from build123d import *

# Parameters (mm, degrees)
BOSS_EXTRUDE1_DEPTH = 15
BOSS_EXTRUDE2_START = 15
BOSS_EXTRUDE2_DEPTH = 3.048
BOSS_EXTRUDE3_START = -15
BOSS_EXTRUDE3_DEPTH = 3.048
SKETCH2_R           = 1.905
CUT_EXTRUDE1_DEPTH  = 46
SKETCH3_R           = 3.5
CUT_EXTRUDE2_DEPTH  = 46


with BuildPart() as part:
    # Sketch1 → Boss-Extrude1 (new, symmetric)
    with BuildSketch(Plane.XY):
        Polygon((-3.048, -30), (0, -30), (0, 0), (-30, 0), (-30, -3.048), (-3.048, -3.048), align=None)
    extrude(amount=BOSS_EXTRUDE1_DEPTH, both=True)

    # Sketch1<3> → Boss-Extrude2 (add)
    with BuildSketch(Plane.XY.offset(BOSS_EXTRUDE2_START)):
        Polygon((-3.048, -30), (-30, -3.048), (-3.048, -3.048), align=None)
    extrude(amount=-BOSS_EXTRUDE2_DEPTH)

    # Sketch1<4> → Boss-Extrude3 (add)
    with BuildSketch(Plane.XY.offset(BOSS_EXTRUDE3_START)):
        Polygon((-3.048, -30), (-30, -3.048), (-3.048, -3.048), align=None)
    extrude(amount=BOSS_EXTRUDE3_DEPTH)

    # Sketch2 → Cut-Extrude1 (cut, through all)
    with BuildSketch(Plane(origin=(0, 0, 0), x_dir=(1, 0, 0), z_dir=(0, 1, 0))):
        with Locations(Location((-15, 0, 0), (0, 0, 270))):
            Circle(SKETCH2_R)
    extrude(amount=-CUT_EXTRUDE1_DEPTH, mode=Mode.SUBTRACT)

    # Sketch3 → Cut-Extrude2 (cut, through all)
    with BuildSketch(Plane(origin=(0, 0, 0), x_dir=(0, 0, -1), z_dir=(1, 0, 0))):
        with Locations((0, -15)):
            Circle(SKETCH3_R)
    extrude(amount=-CUT_EXTRUDE2_DEPTH, mode=Mode.SUBTRACT)


solid = part.part
For this review, take the finished solid that the model builds, in its own axes (mm). A direction names the side the tool comes from. Give positions to 0.01 mm unless a question says otherwise; leave off trailing zeros. Loops run counter-clockwise (first coordinate to the right, second up) from the corner with the lowest first, then second, coordinate; pieces in that order, holes last. Notation, with made-up numbers: (-4.75, -15) -> (11.25, -15) arc R23 cw to (11.25, 19) -> close; hole circle Ø4 at (-21, 64.5). An arc over 180 degrees is marked (long way). One line per question, with ' | ' between items.
1) We need section B-B (y = -12.25). Write out the cut boundary in (x, z), plus the area to 3 significant figures.
Resolved:
outline: (-20.8, -15) -> (0, -15) -> (0, -2.17) -> (-3.05, -2.17) -> (-3.05, -11.95) -> (-20.8, -11.95) -> close; (-20.8, 11.95) -> (-3.05, 11.95) -> (-3.05, 2.17) -> (0, 2.17) -> (0, 15) -> (-20.8, 15) -> close | area: 186 mm2
2) Insertion check: pin 1 Ø12 at (y, z) = (-10.5, -3) entering from -X; pin 2 Ø1 at (x, z) = (-4.5, -4.5) entering from -Y. Each pin has a flat end and moves straight along its axis. Give the tip position at first contact, or say it passes through.
Resolved:
pin 1: stops at x = -3.05 | pin 2: stops at y = -3.05
3) For faces 1 (the flat face through (-16.34, -16.71, 13.5)), 2 (the flat face through (-13, -13, -11.952)), list the 3-axis set-ups (+Z, -Z, +X, -X, +Y, -Y) from which the entire face can be reached by the end or side of a thin tool; tool diameter is ignored.
Resolved:
face 1: +Z, -Z, -X, -Y | face 2: -X, -Y
4) We need section D-D (z = -6.5). Write out the cut boundary in (x, y).
Resolved:
outline: (-30, -3.05) -> (-3.05, -3.05) -> (-3.05, -30) -> (0, -30) -> (0, 0) -> (-30, 0) -> close
5) To check wall thickness, follow probe 1 along Z at (x, y) = (-4.75, -8); probe 2 along Y at (x, z) = (-1.5, 0); probe 3 along X at (y, z) = (-1.95, 0) (3 decimals). State the ranges of each line that lie inside material, in increasing order.
Resolved:
probe 1: z = -15 to -11.95, 11.95 to 15 | probe 2: y = -30 to -18.5, -11.5 to 0 | probe 3: x = -30 to -16.905, -13.095 to 0
6) We need section A-A (z = 0). Write out the cut boundary in (x, y) (3 decimals).
Resolved:
outline: (-30, -3.048) -> (-16.905, -3.048) -> (-16.905, 0) -> (-30, 0) -> close; (-13.095, -3.048) -> (-3.048, -3.048) -> (-3.048, -11.5) -> (0, -11.5) -> (0, 0) -> (-13.095, 0) -> close; (-3.048, -30) -> (0, -30) -> (0, -18.5) -> (-3.048, -18.5) -> close
7) We need section C-C (x = -15). Write out the cut boundary in (y, z) (3 decimals).
Resolved:
outline: (-18.048, -15) -> (0, -15) -> (0, -1.905) -> (-3.048, -1.905) -> (-3.048, -11.952) -> (-18.048, -11.952) -> close; (-18.048, 11.952) -> (-3.048, 11.952) -> (-3.048, 1.905) -> (0, 1.905) -> (0, 15) -> (-18.048, 15) -> close
8) The part is to be moulded in two halves that separate along Z. For faces 3 (the flat face through (-11, -11, -15)), 4 (the flat face through (-30, -2, 0)), 5 (the cylindrical face through (-1.503, -18.417, 0.759)), say which applies: +Z half, -Z half, draft (parallel to the pull), parting line (faces both ways), or undercut.
Resolved:
face 3: -Z half | face 4: draft | face 5: undercut
